Geometry: final body of the model. Coordinates: model frame, mm. Coordinates: 2 decimals unless noted, no trailing zeros. Write each loop counter-clockwise with the first axis right and the second up, starting at its lowest first coordinate (ties: lowest second). Pieces come first, ordered by that corner, then holes. Notation, with made-up numbers: (-12.5, 3.5) -> (16.5, 3.5) arc R28 ccw to (16.5, 33.5) -> close; hole circle Ø7 at (41, 1). An arc over 180 degrees is marked (long way). One line per item, written item: value.
```python
from build123d import *

# Parameters (mm, degrees)
F0_R     = 2.5
F1_DEPTH = 5


with BuildPart() as f1:
    # F0 (on Front) → F1 (new body)
    with BuildSketch(Plane.XZ):
        Polygon((-55, -75), (55, -75), (55, 75), (0, 75), (-55, 75), (-55, 38.300177), align=None)
        with Locations((-40, -55)):
            Circle(F0_R, mode=Mode.SUBTRACT)
        with Locations((-40, -9.5)):
            Circle(F0_R, mode=Mode.SUBTRACT)
        with Locations((0, -55)):
            Circle(F0_R, mode=Mode.SUBTRACT)
        with Locations((40, -55)):
            Circle(F0_R, mode=Mode.SUBTRACT)
        with Locations((0, -9.5)):
            Circle(F0_R, mode=Mode.SUBTRACT)
        with Locations((40, -9.5)):
            Circle(F0_R, mode=Mode.SUBTRACT)
        with Locations((-40, 28)):
            Circle(F0_R, mode=Mode.SUBTRACT)
        with Locations((0, 28)):
            Circle(F0_R, mode=Mode.SUBTRACT)
        with Locations((40, 28)):
            Circle(F0_R, mode=Mode.SUBTRACT)
    extrude(amount=F1_DEPTH)


solid = f1.part
```
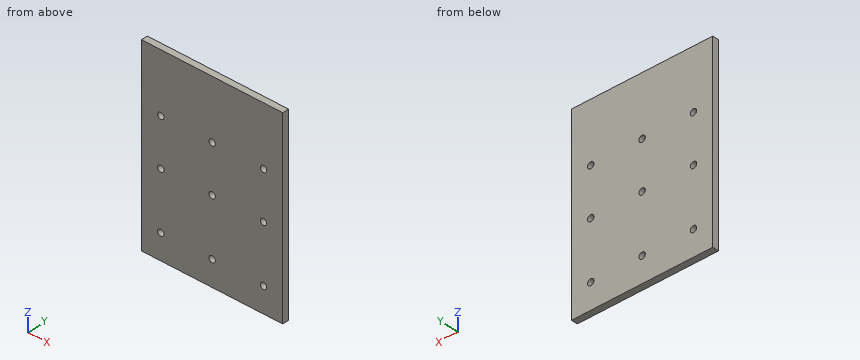
(1) Line query: line 1 (Z direction, x = 40, y = -2.7); line 2 (X direction, y = -2.5, z = -8). Output: solid intervals per line, ascending. Write a range as [from, to].
Responses:
line 1: z = [-75, -57.5], [-52.5, -12], [-7, 25.5], [30.5, 75]
line 2: x = [-55, -42], [-38, -2], [2, 38], [42, 55]
(2) Section A-A (z = -9.5). Return the cut outline in (x, y).
Responses:
outline: (-55, -5) -> (-42.5, -5) -> (-42.5, 0) -> (-55, 0) -> close; (-37.5, -5) -> (-2.5, -5) -> (-2.5, 0) -> (-37.5, 0) -> close; (2.5, -5) -> (37.5, -5) -> (37.5, 0) -> (2.5, 0) -> close; (42.5, -5) -> (55, -5) -> (55, 0) -> (42.5, 0) -> close
(3) First-contact query: pin 1 (4 mm diameter, centred on x = -40, z = 28, fed in from -Y); pin 2 (6.5 mm diameter, centred on x = 40, z = -9.5, fed in from +Y). Flat tips, straight axial feed; report the tip coordinate or a pass-through.
Responses:
pin 1: passes through
pin 2: stops at y = 0
(4) Section B-B (x = 40). Return the cut outline in (y, z).
Responses:
outline: (-5, -75) -> (0, -75) -> (0, -57.5) -> (-5, -57.5) -> close; (-5, -52.5) -> (0, -52.5) -> (0, -12) -> (-5, -12) -> close; (-5, -7) -> (0, -7) -> (0, 25.5) -> (-5, 25.5) -> close; (-5, 30.5) -> (0, 30.5) -> (0, 75) -> (-5, 75) -> close
